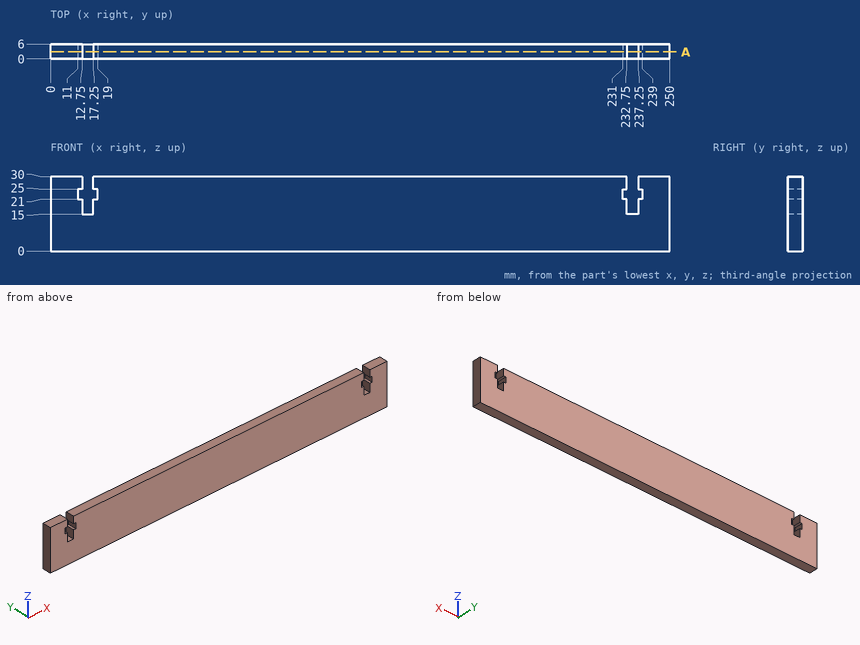
For this review, use the dimensioned drawing (mm, ordinates from the lowest corner) and the shaded views. Coordinates: 2 decimals unless noted, no trailing zeros. Order: outer loops, then holes, each group sorted by start corner. A loop starts at its lowest first (then second) coordinate and runs counter-clockwise, first axis right, second up. Notation, with made-up numbers: (89, 52.25) - (113, 52.25) arc R19 ccw to (113, 76.25) - close; hole circle Ø8 at (-38, 74.25). An arc over 180 degrees is marked (long way). Answer as a JSON object with one key per item and string values. Group by question number.
1. For probe 1 along X at (y, z) = (5.05, 15.5); probe 2 along X at (y, z) = (1.1, 21.25), list the stretches that pass through material, from the lowest coordinate up.
2. We need section A-A on y = 2.8. State the section outline as (x, z) points.
3. Clearance check with flat-ended pins moving along their axes: P1, Ø1.2, axis at y = 2.5, z = 23, coming from the -X side; P2, Ø2, axis at x = 14.5, y = 3.5, coming from the +Z side. State where each tip first meets the part, or that it passes through.
Final values:
{
 "1": {"probe 1": "0 to 12.75, 17.25 to 232.75, 237.25 to 250", "probe 2": "0 to 11, 19 to 231, 239 to 250"},
 "2": {"outline": "(0, 0) - (250, 0) - (250, 30) - (237.25, 30) - (237.25, 25) - (239, 25) - (239, 21) - (237.25, 21) - (237.25, 15) - (232.75, 15) - (232.75, 21) - (231, 21) - (231, 25) - (232.75, 25) - (232.75, 30) - (17.25, 30) - (17.25, 25) - (19, 25) - (19, 21) - (17.25, 21) - (17.25, 15) - (12.75, 15) - (12.75, 21) - (11, 21) - (11, 25) - (12.75, 25) - (12.75, 30) - (0, 30) - close"},
 "3": {"P1": "x = 0", "P2": "z = 15"}
}
